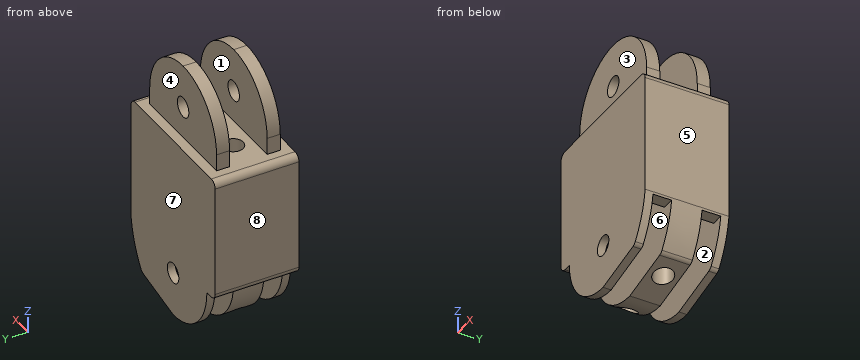
from build123d import *

# Parameters (mm, degrees)
SKETCH2_W             = 17.554431489
SKETCH2_H             = 1.95
BOSS_EXTRUDE1_DEPTH   = 8.75
BOSS_EXTRUDE1_2_DEPTH = 8.75
CUT_EXTRUDE1_DEPTH    = 26.518349076
SKETCH4_W             = 22.027215745
SKETCH4_H             = 12.505427167
BOSS_EXTRUDE2_DEPTH   = 30
SKETCH5_R             = 1.5
CUT_EXTRUDE2_DEPTH    = 12
SKETCH6_W             = 22.027215745
SKETCH6_H             = 12.505427167
SKETCH6_W_2           = 17.554431489
SKETCH6_H_2           = 1.95
CUT_EXTRUDE3_DEPTH    = 2.5
SKETCH7_R             = 1.5
CUT_EXTRUDE4_DEPTH    = 13
SKETCH8_R             = 1.5
CUT_EXTRUDE5_DEPTH    = 28
FILLET3_R             = 1
SKETCH9_W             = 22.022981174
SKETCH9_H             = 2.796352896
SKETCH9_H_2           = 2.782097604
CUT_EXTRUDE6_DEPTH    = 11
SKETCH10_W            = 17.952287352
SKETCH10_H            = 2.796352896
SKETCH10_H_2          = 2.782097604
CUT_EXTRUDE7_DEPTH    = 5


with BuildPart() as part:
    # Sketch2 → Boss-Extrude1 (new body)
    with BuildSketch(Plane.XY):
        with Locations((-13.228930986, -27.845183414)):
            Rectangle(SKETCH2_W, SKETCH2_H)
    extrude(amount=BOSS_EXTRUDE1_DEPTH)


with BuildPart() as body_2:
    # Sketch2 → Boss-Extrude1 2 (new body)
    with BuildSketch(Plane.XY):
        with Locations((-13.228930986, -20.289756247)):
            Rectangle(SKETCH2_W, SKETCH2_H)
    extrude(amount=BOSS_EXTRUDE1_2_DEPTH)


with BuildPart() as cut_extrude1_tool:
    # Sketch3 → Cut-Extrude1 (new, through all)
    with BuildSketch(Plane(origin=(0, -19.314756247, 0), x_dir=(1, 0, 0), z_dir=(0, 1, 0))):
        with BuildLine():
            ThreePointArc((-13.228930986, -8.75), (-7.041746651, -6.187184335), (-4.478930986, 0))
            add(Edge.make_bspline(
                [(-4.478930986, 0), (1.138349918, -4.151657709), (-4.451715242, -8.75)],
                knots=[0, 0, 0, 1, 1, 1], degree=2))
            add(Edge.make_bspline(
                [(-22.006146731, -8.75), (-13.228930986, -12.473510392), (-4.451715242, -8.75)],
                knots=[0, 0, 0, 1, 1, 1], degree=2))
            add(Edge.make_bspline(
                [(-21.978930986, 0), (-25.926969228, -4.242865138), (-22.006146731, -8.75)],
                knots=[0, 0, 0, 1, 1, 1], degree=2))
            ThreePointArc((-21.978930986, 0), (-19.416115322, -6.187184335), (-13.228930986, -8.75))
        make_face()
    extrude(amount=-CUT_EXTRUDE1_DEPTH)


with BuildPart() as part_1:
    add(part.part)

    # Cut-Extrude1: cut by cut_extrude1_tool
    add(cut_extrude1_tool.part, mode=Mode.SUBTRACT)



with BuildPart() as body_2_1:
    add(body_2.part)

    # Cut-Extrude1: cut by cut_extrude1_tool
    add(cut_extrude1_tool.part, mode=Mode.SUBTRACT)


with BuildPart() as part_2:
    add(part_1.part)

    add(body_2_1.part)  # Boss-Extrude2 merges body 2
    # Sketch4 → Boss-Extrude2 (add)
    with BuildSketch(Plane(origin=(0, 0, 0), x_dir=(-1, 0, 0), z_dir=(0, 0, -1))):
        with Locations((13.242538859, -24.067469831)):
            Rectangle(SKETCH4_W, SKETCH4_H)
    extrude(amount=BOSS_EXTRUDE2_DEPTH)

    # Sketch5 → Cut-Extrude2 (cut)
    with BuildSketch(Plane(origin=(0, -19.314756247, 0), x_dir=(1, 0, 0), z_dir=(0, 1, 0))):
        with Locations(Location((-13.228930986, -2.25, 0), (0, 0, 270))):
            Circle(SKETCH5_R)
    extrude(amount=-CUT_EXTRUDE2_DEPTH, mode=Mode.SUBTRACT)

    # Sketch6 → Cut-Extrude3 (cut)
    with BuildSketch(Plane.XY):
        with Locations((-13.242538859, -24.067469831)):
            Rectangle(SKETCH6_W, SKETCH6_H)
        with Locations((-13.228930986, -27.845183414)):
            Rectangle(SKETCH6_W_2, SKETCH6_H_2, mode=Mode.SUBTRACT)
        with Locations((-13.228930986, -20.289756247)):
            Rectangle(SKETCH6_W_2, SKETCH6_H_2, mode=Mode.SUBTRACT)
    extrude(amount=-CUT_EXTRUDE3_DEPTH, mode=Mode.SUBTRACT)

    # Sketch7 → Cut-Extrude4 (cut)
    with BuildSketch(Plane(origin=(0, -17.814756247, 0), x_dir=(1, 0, 0), z_dir=(0, 1, 0))):
        with Locations(Location((-13.242538859, 23.405672985, 0), (0, 0, 270))):
            Circle(SKETCH7_R)
        with BuildLine():
            Line((-22.086865874, 21.155672985), (-24.256146731, 21.155672985))
            add(Edge.make_bspline(
                [(-2.228930986, 21.155672985), (11.471530889, 27.189710441), (-11.765166974, 53.431279988), (-37.007876173, 21.523583672), (-24.256146731, 21.155672985)],
                knots=[0, 0, 0, 0, 0.52011282, 1, 1, 1, 1], degree=3))
            add(Edge.make_bspline(
                [(-5.046294073, 28.201654423), (-2.731488374, 25.068620188), (-2.228930986, 21.155672985)],
                knots=[0, 0, 0, 1, 1, 1], degree=2))
            Line((-5.046294073, 28.201654423), (-13.242538859, 30))
            ThreePointArc((-13.242538859, 30), (-19.496422466, 27.409556592), (-22.086865874, 21.155672985))
        make_face()
    extrude(amount=-CUT_EXTRUDE4_DEPTH, mode=Mode.SUBTRACT)

    # Sketch8 → Cut-Extrude5 (cut)
    with BuildSketch(Plane.XY.offset(-2.5)):
        with Locations((-18.011106811, -24.06746983)):
            Circle(SKETCH8_R)
        with Locations((-8.473970906, -24.06746983)):
            Circle(SKETCH8_R)
    extrude(amount=-CUT_EXTRUDE5_DEPTH, mode=Mode.SUBTRACT)

    # Fillet3
    fillet3_edges = [part_2.edges().sort_by_distance(p)[0] for p in [
        (-24.256146731, -24.06746983, -2.5),
        (-24.256146731, -24.06746983, -21.155672985),
        (-2.228930986, -24.06746983, -2.5),
        (-5.046294073, -24.06746983, -28.201654423),
    ]]
    fillet(fillet3_edges, radius=FILLET3_R)

    # Sketch9 → Cut-Extrude6 (cut)
    with BuildSketch(Plane.XY.offset(-32.5)):
        with Locations((-13.24253886, -20.400707387)):
            Rectangle(SKETCH9_W, SKETCH9_H)
        with Locations((-13.24253886, -27.727104636)):
            Rectangle(SKETCH9_W, SKETCH9_H_2)
    extrude(amount=CUT_EXTRUDE6_DEPTH, mode=Mode.SUBTRACT)

    # Sketch10 → Cut-Extrude7 (cut)
    with BuildSketch(Plane(origin=(0, 0, -21.5), x_dir=(-1, 0, 0), z_dir=(0, 0, -1))):
        with Locations((13.104016993, -20.400707387)):
            Rectangle(SKETCH10_W, SKETCH10_H)
        with Locations((13.104016993, -27.727104636)):
            Rectangle(SKETCH10_W, SKETCH10_H_2)
    extrude(amount=-CUT_EXTRUDE7_DEPTH, mode=Mode.SUBTRACT)


solid = part_2.part
Part model, mm, in its own coordinate system. Face numbers are marked on the shaded views. A direction names the side the tool comes from. Give positions to 0.01 mm unless a question says otherwise; leave off trailing zeros. Write each loop counter-clockwise with the first axis right and the second up, starting at its lowest first coordinate (ties: lowest second). Pieces come first, ordered by that corner, then holes.
1) Cut at D-D on x = -15.5. Write the cut outline in (y, z), then the cut area to 3 significant figures.
Resolved:
outline: (-30.32, -29.71) - (-29.12, -29.71) - (-29.12, -16.5) - (-26.34, -16.5) - (-26.34, -29.71) - (-21.8, -29.71) - (-21.8, -16.5) - (-19, -16.5) - (-19, -29.71) - (-17.81, -29.71) - (-17.81, -2.5) - (-19.31, -2.5) - (-19.31, 8.45) - (-21.26, 8.45) - (-21.26, -2.5) - (-26.87, -2.5) - (-26.87, 8.45) - (-28.82, 8.45) - (-28.82, -2.5) - (-30.32, -2.5) - close
area: 309 mm2
2) Cut at B-B on x = -18. Write the cut outline in (y, z).
Resolved:
outline: (-30.32, -28.61) - (-29.12, -28.61) - (-29.12, -16.5) - (-26.34, -16.5) - (-26.34, -28.61) - (-25.57, -28.61) - (-25.57, -2.5) - (-26.87, -2.5) - (-26.87, 7.33) - (-28.82, 7.33) - (-28.82, -2.5) - (-30.32, -2.5) - close; (-22.57, -28.61) - (-21.8, -28.61) - (-21.8, -16.5) - (-19, -16.5) - (-19, -28.61) - (-17.81, -28.61) - (-17.81, -2.5) - (-19.31, -2.5) - (-19.31, 7.33) - (-21.26, 7.33) - (-21.26, -2.5) - (-22.57, -2.5) - close
3) Which spindle directions (+Z, -Z, +X, -X, +Y, -Y) get a long thin tool onto all of the face, cutting with end or side? Do the marked faces 1, 2, 3 and 4. Say none if no direction does.
Resolved:
face 1: +Z, +X, -X
face 2: -Z
face 3: +Z, +X, -X, -Y
face 4: +Z, +X, -X, +Y
4) Cut at A-A on z = 5. Write the cut outline in (x, y).
Resolved:
outline: (-20.41, -28.82) - (-6.05, -28.82) - (-6.05, -26.87) - (-20.41, -26.87) - close; (-20.41, -21.26) - (-6.05, -21.26) - (-6.05, -19.31) - (-20.41, -19.31) - close
5) Probe L1, parallel to X at y = -24, z = -7.5; L2, parallel to Y at x = -21.25, z = -22; L3, parallel to Y at x = -9.75, z = -19. List the from-to ranges inside material, lowest first.
Resolved:
L1: x = -24.26 to -19.51, -16.51 to -9.97, -6.98 to -2.23
L2: y = -30.32 to -29.12, -26.34 to -21.8, -19 to -17.81
L3: y = -30.32 to -29.12, -26.34 to -24.86, -23.28 to -21.8, -19 to -17.81
6) Cut at C-C on z = -18.5. Write the cut outline in (x, y), then the cut area to 3 significant figures.
Resolved:
outline: (-24.26, -30.32) - (-2.23, -30.32) - (-2.23, -17.81) - (-24.26, -17.81) - close; hole (-22.08, -29.12) - (-4.13, -29.12) - (-4.13, -26.34) - (-22.08, -26.34) - close; hole (-22.08, -21.8) - (-4.13, -21.8) - (-4.13, -19) - (-22.08, -19) - close; hole circle Ø3 at (-18.01, -24.07); hole circle Ø3 at (-8.47, -24.07)
area: 161 mm2
7) Pin check, flat tips, straight feed: pin 1 (3.5 mm diameter, centred on x = -13.23, z = 2.25, fed in from +Y); pin 2 (6 mm diameter, centred on x = -22, y = -25.5, fed in from -Z); pin 3 (0.6 mm diameter, centred on x = -3.5, y = -19.5, fed in from -Z). Stop position of each tip, or through.
Resolved:
pin 1: stops at y = -19.31
pin 2: stops at z = -27.87
pin 3: stops at z = -21.5
8) Two-plate mould, pull along X, no slides. Class the marked faces 5, 6, 7 and 8: released by +X, released by -X, zero draft, split by the parting line, or undercut.
Resolved:
face 5: released by +X
face 6: undercut
face 7: zero draft
face 8: released by -X
